from build123d import *

# Parameters (mm, degrees)
SKETCH1_W           = 71.5
SKETCH1_H           = 38.5
BOSS_EXTRUDE1_DEPTH = 29.5
SKETCH1_4_W         = 65.5
SKETCH1_4_H         = 32.5
CUT_EXTRUDE1_DEPTH  = 27
SKETCH3_W           = 6
SKETCH3_H           = 25.5
CUT_EXTRUDE2_DEPTH  = 29
BOSS_EXTRUDE3_DEPTH = 5
BOSS_EXTRUDE4_DEPTH = 5
BOSS_EXTRUDE5_DEPTH = 5
BOSS_EXTRUDE6_DEPTH = 5
SKETCH5_9_R         = 2.5
CUT_EXTRUDE3_DEPTH  = 15
SKETCH5_10_R        = 2.5
CUT_EXTRUDE4_DEPTH  = 20
SKETCH5_11_R        = 2.5
CUT_EXTRUDE5_DEPTH  = 20
SKETCH5_12_R        = 2.5
CUT_EXTRUDE6_DEPTH  = 20
SKETCH4_W           = 5
SKETCH4_H           = 3.5
CUT_EXTRUDE7_DEPTH  = 63
SKETCH4_3_W         = 5
SKETCH4_3_H         = 3.5
CUT_EXTRUDE8_DEPTH  = 63


with BuildPart() as part:
    # Sketch1 → Boss-Extrude1 (new body)
    with BuildSketch(Plane(origin=(0, 0, 0), x_dir=(1, 0, 0), z_dir=(0, 1, 0))):
        with Locations((35.75, 19.25)):
            Rectangle(SKETCH1_W, SKETCH1_H)
    extrude(amount=-BOSS_EXTRUDE1_DEPTH)

    # Sketch1_4 → Cut-Extrude1 (cut)
    with BuildSketch(Plane(origin=(0, 0, 0), x_dir=(1, 0, 0), z_dir=(0, 1, 0))):
        with Locations((35.75, 19.25)):
            Rectangle(SKETCH1_4_W, SKETCH1_4_H)
    extrude(amount=-CUT_EXTRUDE1_DEPTH, mode=Mode.SUBTRACT)

    # Sketch3 → Cut-Extrude2 (cut)
    with BuildSketch(Plane.ZY):
        with Locations((-7.5, -12.75)):
            Rectangle(SKETCH3_W, SKETCH3_H)
        with Locations((-31, -12.75)):
            Rectangle(SKETCH3_W, SKETCH3_H)
    extrude(amount=-CUT_EXTRUDE2_DEPTH, mode=Mode.SUBTRACT)

    # Sketch5 → Boss-Extrude3 (add)
    with BuildSketch(Plane.XZ.offset(29.5)):
        with BuildLine():
            Line((61.5, 0), (61.5, 5))
            ThreePointArc((61.5, 5), (66.5, 10), (71.5, 5))
            Line((71.5, 5), (71.5, 0))
            Line((71.5, 0), (61.5, 0))
        make_face()
    extrude(amount=-BOSS_EXTRUDE3_DEPTH)

    # Sketch5_5 → Boss-Extrude4 (add)
    with BuildSketch(Plane.XZ.offset(29.5)):
        with BuildLine():
            Line((0, 0), (10, 0))
            Line((10, 0), (10, 5))
            ThreePointArc((10, 5), (5, 10), (0, 5))
            Line((0, 5), (0, 0))
        make_face()
    extrude(amount=-BOSS_EXTRUDE4_DEPTH)

    # Sketch5_7 → Boss-Extrude5 (add)
    with BuildSketch(Plane.XZ.offset(29.5)):
        with BuildLine():
            Line((71.5, -38.5), (71.5, -43.5))
            ThreePointArc((71.5, -43.5), (66.5, -48.5), (61.5, -43.5))
            Line((61.5, -43.5), (61.5, -38.5))
            Line((61.5, -38.5), (71.5, -38.5))
        make_face()
    extrude(amount=-BOSS_EXTRUDE5_DEPTH)

    # Sketch5_8 → Boss-Extrude6 (add)
    with BuildSketch(Plane.XZ.offset(29.5)):
        with BuildLine():
            Line((10, -38.5), (10, -43.5))
            ThreePointArc((10, -43.5), (5, -48.5), (0, -43.5))
            Line((0, -43.5), (0, -38.5))
            Line((0, -38.5), (10, -38.5))
        make_face()
    extrude(amount=-BOSS_EXTRUDE6_DEPTH)

    # Sketch5_9 → Cut-Extrude3 (cut)
    with BuildSketch(Plane.XZ.offset(29.5)):
        with Locations(Location((66.5, 5, 0), (0, 0, 90))):
            Circle(SKETCH5_9_R)
    extrude(amount=-CUT_EXTRUDE3_DEPTH, mode=Mode.SUBTRACT)

    # Sketch5_10 → Cut-Extrude4 (cut)
    with BuildSketch(Plane.XZ.offset(29.5)):
        with Locations(Location((5, 5, 0), (0, 0, 270))):
            Circle(SKETCH5_10_R)
    extrude(amount=-CUT_EXTRUDE4_DEPTH, mode=Mode.SUBTRACT)

    # Sketch5_11 → Cut-Extrude5 (cut)
    with BuildSketch(Plane.XZ.offset(29.5)):
        with Locations(Location((5, -43.5, 0), (0, 0, 90))):
            Circle(SKETCH5_11_R)
    extrude(amount=-CUT_EXTRUDE5_DEPTH, mode=Mode.SUBTRACT)

    # Sketch5_12 → Cut-Extrude6 (cut)
    with BuildSketch(Plane.XZ.offset(29.5)):
        with Locations(Location((66.5, -43.5, 0), (0, 0, 270))):
            Circle(SKETCH5_12_R)
    extrude(amount=-CUT_EXTRUDE6_DEPTH, mode=Mode.SUBTRACT)

    # Sketch4 → Cut-Extrude7 (cut)
    with BuildSketch(Plane(origin=(0, 0, -38.5), x_dir=(-1, 0, 0), z_dir=(0, 0, -1))):
        with Locations((-62.806579946, -3.25)):
            Rectangle(SKETCH4_W, SKETCH4_H)
    extrude(amount=-CUT_EXTRUDE7_DEPTH, mode=Mode.SUBTRACT)

    # Sketch4_3 → Cut-Extrude8 (cut)
    with BuildSketch(Plane(origin=(0, 0, -38.5), x_dir=(-1, 0, 0), z_dir=(0, 0, -1))):
        with Locations((-8.693420054, -3.25)):
            Rectangle(SKETCH4_3_W, SKETCH4_3_H)
    extrude(amount=-CUT_EXTRUDE8_DEPTH, mode=Mode.SUBTRACT)


solid = part.part
Geometry: final body of the model. Coordinates: model frame, mm. A direction names the side the tool comes from. Round coordinates to 2 decimals unless told otherwise and drop trailing zeros. Order: outer loops, then holes, each group sorted by start corner. A loop starts at its lowest first (then second) coordinate and runs counter-clockwise, first axis right, second up. Notation, with made-up numbers: (34.25, 49.25) -> (76.25, 49.25) arc R22 cw to (76.25, 56.25) -> close; hole circle Ø6 at (14.25, -12). An arc over 180 degrees is marked (long way). Put each result on its own line as item: value. Start each with the question number.
Q1. Line query: probe 1 along X at (y, z) = (-25.6, 5); probe 2 along Z at (x, y) = (43, -6); probe 3 along Y at (x, z) = (61.5, -38). Output: solid intervals per line, ascending.
Q2. Section A-A on y = -18.5. Return the cut outline in (x, z), and give its area (3 significant figures).
Q3. First-contact query: pin 1 (5 mm diameter, centred on x = 66.5, z = 6, fed in from +Y); pin 2 (4.5 mm diameter, centred on x = 66.5, z = 5, fed in from -Y); pin 3 (8 mm diameter, centred on x = 29.5, z = -30, fed in from +Y); pin 4 (10 mm diameter, centred on x = 45, y = -14, fed in from -Z). Flat tips, straight axial feed; report the tip coordinate or a pass-through.
Q4. Section C-C on z = -33. Return the cut outline in (x, y).
Q5. Pull-direction query (Z, two-part tool) for faces 1 (the flat face through (11.193, -3, -2)), 2 (the flat face through (35, -27, -19)); classes: +Z half, -Z half, draft (parallel to the pull), parting line (faces both ways), or undercut.
Q6. Section B-B on x = 5. Return the cut outline in (y, z), and give its area (3 significant figures).
Q7. Section D-D on x = 48.5. Return the cut outline in (y, z), and give its area (3 significant figures).
Q8. Reachability of faces 3 (the flat face through (1, -25.5, -8)), 4 (the flat face through (10, -27, 2)), 5 (the flat face through (68.5, -13, -19)), 6 (the flat face through (9, -1.5, -2)) from +Z, -Z, +X, -X, +Y, -Y: full face, straight path, thin tool, end or side. Return the list, or none.
Ans:
1. probe 1: x = 0 to 2.5, 7.5 to 10, 61.5 to 64, 69 to 71.5
1. probe 2: z = -38.5 to -35.5, -3 to 0
1. probe 3: y = -29.5 to -5, -1.5 to 0
2. outline: (0, -38.5) -> (71.5, -38.5) -> (71.5, 0) -> (0, 0) -> (0, -4.5) -> (3, -4.5) -> (3, -3) -> (68.5, -3) -> (68.5, -35.5) -> (3, -35.5) -> (3, -34) -> (0, -34) -> close; (0, -28) -> (3, -28) -> (3, -10.5) -> (0, -10.5) -> close
2. area: 588 mm2
3. pin 1: stops at y = -24.5
3. pin 2: passes through
3. pin 3: stops at y = -27
3. pin 4: stops at z = -38.5
4. outline: (0, -29.5) -> (71.5, -29.5) -> (71.5, 0) -> (68.5, 0) -> (68.5, -27) -> (3, -27) -> (3, -25.5) -> (0, -25.5) -> close
5. face 1: draft
5. face 2: undercut
6. outline: (-29.5, -48.5) -> (-24.5, -48.5) -> (-24.5, -46) -> (-29.5, -46) -> close; (-29.5, -41) -> (-24.5, -41) -> (-24.5, -38.5) -> (0, -38.5) -> (0, -35.5) -> (-27, -35.5) -> (-27, -3) -> (0, -3) -> (0, 0) -> (-24.5, 0) -> (-24.5, 2.5) -> (-29.5, 2.5) -> close; (-29.5, 7.5) -> (-24.5, 7.5) -> (-24.5, 10) -> (-29.5, 10) -> close
6. area: 308 mm2
7. outline: (-29.5, -38.5) -> (0, -38.5) -> (0, -35.5) -> (-27, -35.5) -> (-27, -3) -> (0, -3) -> (0, 0) -> (-29.5, 0) -> close
7. area: 258 mm2
8. face 3: -X, +Y
8. face 4: +Z, +Y, -Y
8. face 5: +Y
8. face 6: +Z, -Z
